Study the drawing (mm; zero at the part's minimum x, y, z) and answer. Coordinates: 2 decimals unless noted, no trailing zeros. Order: outer loops, then holes, each group sorted by start corner. A loop starts at its lowest first (then second) coordinate and runs counter-clockwise, first axis right, second up.
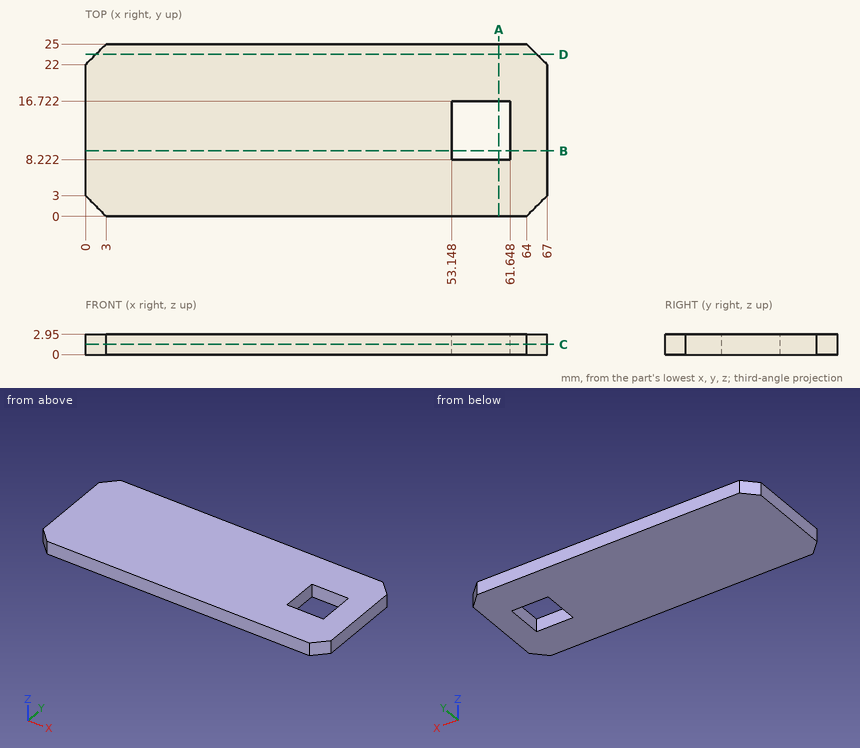
1) Straight lines are drawn through the part: line 1 (X direction, y = 13, z = 0.85); line 2 (Y direction, x = 57, z = 2.75); line 3 (X direction, y = 22.75, z = 0.5). For each, find the intervals that lie inside material, in ascending order.
A:
line 1: x = 0 to 53.15, 61.65 to 67
line 2: y = 0 to 8.22, 16.72 to 25
line 3: x = 0.75 to 66.25
2) A cutting plane is placed at B-B, the plane y = 9.5. Determine the outline of the cut face in (x, z).
A:
outline: (0, 0) - (53.15, 0) - (53.15, 2.95) - (0, 2.95) - close; (61.65, 0) - (67, 0) - (67, 2.95) - (61.65, 2.95) - close
3) A cutting plane is placed at C-C, the plane z = 1.5. Determine the outline of the cut face in (x, y), and give its area (3 significant figures).
A:
outline: (0, 3) - (3, 0) - (64, 0) - (67, 3) - (67, 22) - (64, 25) - (3, 25) - (0, 22) - close; hole (53.15, 8.22) - (61.65, 8.22) - (61.65, 16.72) - (53.15, 16.72) - close
area: 1,580 mm2
4) A cutting plane is placed at A-A, the plane x = 60. Determine the outline of the cut face in (y, z).
A:
outline: (0, 0) - (8.22, 0) - (8.22, 2.95) - (0, 2.95) - close; (16.72, 0) - (25, 0) - (25, 2.95) - (16.72, 2.95) - close
5) A cutting plane is placed at D-D, the plane y = 23.5. Determine the outline of the cut face in (x, z).
A:
outline: (1.5, 0) - (65.5, 0) - (65.5, 2.95) - (1.5, 2.95) - close
